Read the model definition and answer for the solid it produces. Units are mm, in the model's axes. Coordinates: 2 decimals unless noted, no trailing zeros. Write each loop counter-clockwise with the first axis right and the second up, starting at its lowest first coordinate (ties: lowest second). Pieces come first, ordered by that corner, then holes. Notation, with made-up numbers: (88, 78.25) -> (119, 78.25) arc R27 ccw to (119, 116.25) -> close; hole circle Ø8 at (2.25, -26). An arc over 180 degrees is marked (long way). Return JSON: item names as keys, results as strings.
from build123d import *

# Parameters (mm, degrees)
F0_W     = 550
F0_H     = 452
F0_W_2   = 445
F0_H_2   = 345
F1_DEPTH = 22.5
F2_SIZE2 = 5
F2_SIZE  = 18
F3_SIZE2 = 12
F3_SIZE  = 8


with BuildPart() as f1:
    # F0 (on Front) → F1 (new body, symmetric)
    with BuildSketch(Plane.XZ):
        Rectangle(F0_W, F0_H)
        Rectangle(F0_W_2, F0_H_2, mode=Mode.SUBTRACT)
    extrude(amount=F1_DEPTH, both=True)

    # F2
    f2_edges = [f1.edges().sort_by_distance(p)[0] for p in [
        (0, 22.5, -172.5),
        (222.5, 22.5, 0),
        (-222.5, 22.5, 0),
        (0, 22.5, 172.5),
    ]]
    chamfer(f2_edges, length=F2_SIZE, length2=F2_SIZE2)

    # F3
    f3_edges = [f1.edges().sort_by_distance(p)[0] for p in [
        (0, -22.5, -172.5),
        (-222.5, -22.5, 0),
        (222.5, -22.5, 0),
        (0, -22.5, 172.5),
    ]]
    f3_side = f1.faces().sort_by_distance((0, -22.5, 218.880983))[0]
    chamfer(f3_edges, length=F3_SIZE, length2=F3_SIZE2, reference=f3_side)


solid = f1.part
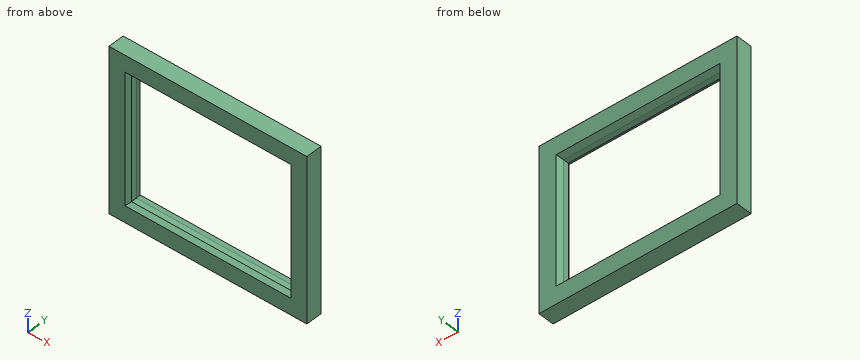
1. The part is cut by section C-C (z = -78). Determine the outline of the cut face in (x, y), then the cut area to 3 significant figures.
Taken from the geometry:
{"outline": "(-275, -22.5) -> (-230.5, -22.5) -> (-222.5, -10.5) -> (-222.5, 4.5) -> (-227.5, 22.5) -> (-275, 22.5) -> close; (222.5, -10.5) -> (230.5, -22.5) -> (275, -22.5) -> (275, 22.5) -> (227.5, 22.5) -> (222.5, 4.5) -> close", "area": "4,540 mm2"}
2. The part is cut by section B-B (y = -4). Determine the outline of the cut face in (x, z).
Taken from the geometry:
{"outline": "(-275, -226) -> (275, -226) -> (275, 226) -> (-275, 226) -> close; hole (-222.5, -172.5) -> (222.5, -172.5) -> (222.5, 172.5) -> (-222.5, 172.5) -> close"}
3. Consider L1, parallel to X at y = 4, z = -68.5; L2, parallel to Z at x = 141, y = -2; L3, parallel to X at y = -12, z = 151. Determine where each line is inside the solid, lowest interval first.
Taken from the geometry:
{"L1": "x = -275 to -222.5, 222.5 to 275", "L2": "z = -226 to -172.5, 172.5 to 226", "L3": "x = -275 to -223.5, 223.5 to 275"}
4. The part is cut by section A-A (x = 110.5). Determine the outline of the cut face in (y, z).
Taken from the geometry:
{"outline": "(-22.5, -226) -> (22.5, -226) -> (22.5, -177.5) -> (4.5, -172.5) -> (-10.5, -172.5) -> (-22.5, -180.5) -> close; (-22.5, 180.5) -> (-10.5, 172.5) -> (4.5, 172.5) -> (22.5, 177.5) -> (22.5, 226) -> (-22.5, 226) -> close"}
